```python
from build123d import *

# Parameters (mm, degrees)
SKETCH1_R      = 2.5527
FINALCUT_DEPTH = 101.6


with BuildPart() as part:
    # Sketch1 → FinalCut (new body)
    with BuildSketch(Plane.XY):
        with BuildLine():
            Line((-4.7498, 0), (-4.7498, 3.187235435))
            Line((-4.7498, 3.187235435), (-10.3632, 8.800635435))
            Line((-10.3632, 8.800635435), (-10.3632, 3.2258))
            Line((-10.3632, 3.2258), (-12.7, 3.2258))
            Line((-12.7, 3.2258), (-12.7, 10.668))
            ThreePointArc((-12.7, 10.668), (-12.104840979, 12.104840979), (-10.668, 12.7))
            Line((-10.668, 12.7), (-3.2258, 12.7))
            Line((-3.2258, 12.7), (-3.2258, 10.3632))
            Line((-3.2258, 10.3632), (-8.800635435, 10.3632))
            Line((-8.800635435, 10.3632), (-3.187235435, 4.7498))
            Line((-3.187235435, 4.7498), (0, 4.7498))
            Line((0, 4.7498), (3.187235435, 4.7498))
            Line((3.187235435, 4.7498), (8.800635435, 10.3632))
            Line((8.800635435, 10.3632), (3.2258, 10.3632))
            Line((3.2258, 10.3632), (3.2258, 12.7))
            Line((3.2258, 12.7), (10.668, 12.7))
            ThreePointArc((10.668, 12.7), (12.104840979, 12.104840979), (12.7, 10.668))
            Line((12.7, 10.668), (12.7, 3.2258))
            Line((12.7, 3.2258), (10.3632, 3.2258))
            Line((10.3632, 3.2258), (10.3632, 8.800635435))
            Line((10.3632, 8.800635435), (4.7498, 3.187235435))
            Line((4.7498, 3.187235435), (4.7498, 0))
            Line((4.7498, 0), (4.7498, -3.187235435))
            Line((4.7498, -3.187235435), (10.3632, -8.800635435))
            Line((10.3632, -8.800635435), (10.3632, -3.2258))
            Line((10.3632, -3.2258), (12.7, -3.2258))
            Line((12.7, -3.2258), (12.7, -10.668))
            ThreePointArc((12.7, -10.668), (12.104840979, -12.104840979), (10.668, -12.7))
            Line((10.668, -12.7), (3.2258, -12.7))
            Line((3.2258, -12.7), (3.2258, -10.3632))
            Line((3.2258, -10.3632), (8.800635435, -10.3632))
            Line((8.800635435, -10.3632), (3.187235435, -4.7498))
            Line((3.187235435, -4.7498), (0, -4.7498))
            Line((0, -4.7498), (-3.187235435, -4.7498))
            Line((-3.187235435, -4.7498), (-8.800635435, -10.3632))
            Line((-8.800635435, -10.3632), (-3.2258, -10.3632))
            Line((-3.2258, -10.3632), (-3.2258, -12.7))
            Line((-3.2258, -12.7), (-10.668, -12.7))
            ThreePointArc((-10.668, -12.7), (-12.104840979, -12.104840979), (-12.7, -10.668))
            Line((-12.7, -10.668), (-12.7, -3.2258))
            Line((-12.7, -3.2258), (-10.3632, -3.2258))
            Line((-10.3632, -3.2258), (-10.3632, -8.800635435))
            Line((-10.3632, -8.800635435), (-4.7498, -3.187235435))
            Line((-4.7498, -3.187235435), (-4.7498, 0))
        make_face()
        Circle(SKETCH1_R, mode=Mode.SUBTRACT)
    extrude(amount=-FINALCUT_DEPTH)


solid = part.part
```
Verification items for the finished model (mm, model axes). A direction names the side the tool comes from. Round coordinates to 2 decimals unless told otherwise and drop trailing zeros. Write each loop counter-clockwise with the first axis right and the second up, starting at its lowest first coordinate (ties: lowest second). Pieces come first, ordered by that corner, then holes. Notation, with made-up numbers: (51.5, 2.5) -> (61.5, 2.5) arc R22 ccw to (61.5, 16.5) -> close; hole circle Ø7 at (52, 86). An arc over 180 degrees is marked (long way). Write each question's results on one line, items separated by ' | '. Start each with the question number.
1. Cross-section at D-D (x = -6). Enter the section's corners in (y, z).
2. Draft check along Y on faces 5 (the flat face through (-7, -12.7, -50)), 6 (the flat face through (6, -10.363, -50)), 7 (the flat face through (0, 3, -101.6)), 8 (the flat face through (-7, 12.7, -50)). Enter one of: +Y half, -Y half, draft (parallel to the pull), parting line (faces both ways), or undercut.
3. Cross-section at A-A (x = 0). Enter the section's corners in (y, z), then the cut area to 3 significant figures.
4. Cross-section at C-C (y = 7.25). Enter the section's corners in (x, z), then the cut area to 3 significant figures.
5. Material ranges on probe 1 along X at (y, z) = (-3.75, -52); probe 2 along Y at (x, z) = (-8.5, -55.5); probe 3 along Y at (x, z) = (-5.5, -16), recorded low to high. Write a range as from..to.
6. Depth check by flat-ended pin: P1, Ø1.2, axis at x = 12, z = -45.5, coming from the +Y side; P2, Ø1.2, axis at y = 12, z = -32, coming from the -X side; P3, Ø0.7, axis at y = 11.5, z = -58, coming from the +X side; P4, Ø6, axis at x = 2, y = -9, coming from the -Z side. Enter the tip coordinate at first touch or a pass-through.
7. Set-up check for faces 1 (the flat face through (-4.75, 0, -50)), 2 (the flat face through (0, 4.75, -50)), 3 (the flat face through (3.226, -12, -50)), 4 (the flat face through (-7.596, -6.033, -50.089)): record each of +Z, -Z, +X, -X, +Y, -Y from which the full face is reachable in a straight line by a thin tool's end or side.
Solutions:
1) outline: (-12.7, -101.6) -> (-10.36, -101.6) -> (-10.36, 0) -> (-12.7, 0) -> close; (-7.56, -101.6) -> (-4.44, -101.6) -> (-4.44, 0) -> (-7.56, 0) -> close; (4.44, -101.6) -> (7.56, -101.6) -> (7.56, 0) -> (4.44, 0) -> close; (10.36, -101.6) -> (12.7, -101.6) -> (12.7, 0) -> (10.36, 0) -> close
2) face 5: -Y half | face 6: undercut | face 7: draft | face 8: +Y half
3) outline: (-4.75, -101.6) -> (-2.55, -101.6) -> (-2.55, 0) -> (-4.75, 0) -> close; (2.55, -101.6) -> (4.75, -101.6) -> (4.75, 0) -> (2.55, 0) -> close | area: 446 mm2
4) outline: (-12.7, -101.6) -> (-10.36, -101.6) -> (-10.36, 0) -> (-12.7, 0) -> close; (-8.81, -101.6) -> (-5.69, -101.6) -> (-5.69, 0) -> (-8.81, 0) -> close; (5.69, -101.6) -> (8.81, -101.6) -> (8.81, 0) -> (5.69, 0) -> close; (10.36, -101.6) -> (12.7, -101.6) -> (12.7, 0) -> (10.36, 0) -> close | area: 1,110 mm2
5) probe 1: x = -12.7..-10.36, -5.31..5.31, 10.36..12.7 | probe 2: y = -12.7..-10.36, -10.06..-6.94, 6.94..10.06, 10.36..12.7 | probe 3: y = -12.7..-10.36, -7.06..-3.94, 3.94..7.06, 10.36..12.7
6) P1: stops at y = 12.56 | P2: stops at x = -12.56 | P3: stops at x = 12.64 | P4: stops at z = -101.6
7) face 1: +Z, -Z, -X | face 2: +Z, -Z, +Y | face 3: +Z, -Z, -Y | face 4: +Z, -Z
